```python
from build123d import *

# Parameters (mm, degrees)
SKETCH1_W           = 192.0875
SKETCH1_H           = 95.9358
BOSS_EXTRUDE1_DEPTH = 6.35
SKETCH8_R           = 0.635
CUT_EXTRUDE2_DEPTH  = 20.05
SKETCH3_R           = 2.54
SKETCH3_W           = 12.8016
SKETCH3_H           = 27.94
SKETCH3_W_2         = 18.034
SKETCH3_H_2         = 12.7
CUT_EXTRUDE3_DEPTH  = 7.35


with BuildPart() as part:
    # Sketch1 → Boss-Extrude1 (new body)
    with BuildSketch(Plane(origin=(0, 0, 0), x_dir=(1, 0, 0), z_dir=(0, 1, 0))):
        with Locations((96.04375, 47.9679)):
            Rectangle(SKETCH1_W, SKETCH1_H)
    extrude(amount=BOSS_EXTRUDE1_DEPTH)

    # Sketch8 → Cut-Extrude2 (cut, through all)
    with BuildSketch(Plane.XZ.offset(12.7)):
        with Locations((19.05, 5.6642)):
            Circle(SKETCH8_R)
        with Locations((19.05, 18.3642)):
            Circle(SKETCH8_R)
        with Locations((19.05, -70.5358)):
            Circle(SKETCH8_R)
        with Locations((19.05, -83.2358)):
            Circle(SKETCH8_R)
        with Locations((57.15, -52.7558)):
            Circle(SKETCH8_R)
        with Locations((57.15, -14.6558)):
            Circle(SKETCH8_R)
        with Locations((96.2406, -14.6558)):
            Circle(SKETCH8_R)
        with Locations((96.2406, -52.7558)):
            Circle(SKETCH8_R)
        with Locations((107.95, -83.2358)):
            Circle(SKETCH8_R)
        with Locations((107.95, -70.5358)):
            Circle(SKETCH8_R)
        with Locations((107.95, 5.6642)):
            Circle(SKETCH8_R)
        with Locations((107.95, 18.3642)):
            Circle(SKETCH8_R)
    extrude(amount=-CUT_EXTRUDE2_DEPTH, mode=Mode.SUBTRACT)

    # Sketch3 → Cut-Extrude3 (cut, through all)
    with BuildSketch(Plane(origin=(0, 0, 0), x_dir=(-1, 0, 0), z_dir=(0, -1, 0))):
        with Locations((-96.04375, 25.4)):
            Circle(SKETCH3_R)
        with Locations((-96.04375, 70.5358)):
            Circle(SKETCH3_R)
        with BuildLine():
            Line((-11.43, 88.9508), (-11.43, 82.6008))
            ThreePointArc((-11.43, 82.6008), (-12.7, 81.3308), (-13.97, 82.6008))
            Line((-13.97, 82.6008), (-13.97, 88.9508))
            ThreePointArc((-13.97, 88.9508), (-12.7, 90.2208), (-11.43, 88.9508))
        make_face()
        with BuildLine():
            Line((-182.5625, 84.5058), (-176.2125, 84.5058))
            ThreePointArc((-176.2125, 84.5058), (-174.9425, 85.7758), (-176.2125, 87.0458))
            Line((-176.2125, 87.0458), (-182.5625, 87.0458))
            ThreePointArc((-182.5625, 87.0458), (-183.8325, 85.7758), (-182.5625, 84.5058))
        make_face()
        with BuildLine():
            Line((-9.525, 11.43), (-15.875, 11.43))
            ThreePointArc((-15.875, 11.43), (-17.145, 10.16), (-15.875, 8.89))
            Line((-15.875, 8.89), (-9.525, 8.89))
            ThreePointArc((-9.525, 8.89), (-8.255, 10.16), (-9.525, 11.43))
        make_face()
        with BuildLine():
            Line((-5.1054, 16.7894), (-11.4554, 16.7894))
            ThreePointArc((-11.4554, 16.7894), (-12.5222, 17.8562), (-11.4554, 18.923))
            Line((-11.4554, 18.923), (-5.1054, 18.923))
            ThreePointArc((-5.1054, 18.923), (-4.0386, 17.8562), (-5.1054, 16.7894))
        make_face()
        with BuildLine():
            Line((-186.9821, 16.7894), (-180.6321, 16.7894))
            ThreePointArc((-180.6321, 16.7894), (-179.5653, 17.8562), (-180.6321, 18.923))
            Line((-180.6321, 18.923), (-186.9821, 18.923))
            ThreePointArc((-186.9821, 18.923), (-188.0489, 17.8562), (-186.9821, 16.7894))
        make_face()
        with Locations((-172.5803, 49.1998)):
            Rectangle(SKETCH3_W, SKETCH3_H)
        with Locations((-19.5072, 49.1998)):
            Rectangle(SKETCH3_W, SKETCH3_H)
        with BuildLine():
            Line((-186.9821, 79.1464), (-180.6321, 79.1464))
            ThreePointArc((-180.6321, 79.1464), (-179.5653, 78.0796), (-180.6321, 77.0128))
            Line((-180.6321, 77.0128), (-186.9821, 77.0128))
            ThreePointArc((-186.9821, 77.0128), (-188.0489, 78.0796), (-186.9821, 79.1464))
        make_face()
        with Locations((-75.311, 49.1998)):
            Rectangle(SKETCH3_W_2, SKETCH3_H_2)
    extrude(amount=-CUT_EXTRUDE3_DEPTH, mode=Mode.SUBTRACT)


solid = part.part
```
The listing builds one solid part. Answer for the finished solid, in the listing's coordinates (mm). A direction names the side the tool comes from. Give positions to 0.01 mm unless a question says otherwise; leave off trailing zeros. Write each loop counter-clockwise with the first axis right and the second up, starting at its lowest first coordinate (ties: lowest second). Pieces come first, ordered by that corner, then holes. Notation, with made-up numbers: (-9.5, -5.75) -> (14.5, -5.75) arc R21 ccw to (14.5, 3.25) -> close; hole circle Ø5 at (22, 38). An arc over 180 degrees is marked (long way). Write item = value, one per line. Start each with the question number.
1) The part is cut by section C-C, the plane x = 82. Determine the outline of the cut face in (y, z), and give its area (3 significant figures).
2) The part is cut by section D-D, the plane y = 2. Count the separate pieces of the cut face and the enclosed holes in it, and give its area (3 significant figures).
3) The part is cut by section A-A, the plane z = -61. Determine the outline of the cut face in (x, y).
4) Straight lines are drawn through the part: line 1 along X through (y, z) = (1, -58.5); line 2 along X through (y, z) = (3.75, -49.5); line 3 along Z through (x, y) = (168.5, 1.5). For each, find the intervals that lie inside material, in ascending order.
5) Determine the mould class of faces 3 (the face through (13, 3, -11.43)), 4 (the face through (192.088, 3, -47)), 5 (the face through (95, 3, -95.936)) for opening direction X: +X half, -X half, draft (parallel to the pull), parting line (faces both ways), or undercut.
6) Which of the six approach directions +Z, -Z, +X, -X, +Y, -Y give full straight-line access (tool end or side, diameter ignored) to faces 1 (the face through (0, 3, -47)), 2 (the face through (11.43, 3, -86))?
7) The part is cut by section B-B, the plane z = -25.4. Determine the outline of the cut face in (x, y), and give its area (3 significant figures).
Solutions:
q1.outline = (0, -95.94) -> (6.35, -95.94) -> (6.35, -55.55) -> (0, -55.55) -> close; (0, -42.85) -> (6.35, -42.85) -> (6.35, 0) -> (0, 0) -> close
q1.area = 529 mm²
q2.separate_pieces = 1
q2.enclosed_holes = 19
q2.area = 17,300 mm²
q3.outline = (0, 0) -> (13.11, 0) -> (13.11, 6.35) -> (0, 6.35) -> close; (25.91, 0) -> (166.18, 0) -> (166.18, 6.35) -> (25.91, 6.35) -> close; (178.98, 0) -> (192.09, 0) -> (192.09, 6.35) -> (178.98, 6.35) -> close
q4.line_1 = 0 to 13.11, 25.91 to 166.18, 178.98 to 192.09
q4.line_2 = 0 to 13.11, 25.91 to 66.29, 84.33 to 166.18, 178.98 to 192.09
q4.line_3 = -95.94 to -63.17, -35.23 to 0
q5.face_3 = undercut
q5.face_4 = +X half
q5.face_5 = draft
q6.face_1 = +Z, -Z, -X, +Y, -Y
q6.face_2 = +Y, -Y
q7.outline = (0, 0) -> (93.5, 0) -> (93.5, 6.35) -> (0, 6.35) -> close; (98.58, 0) -> (192.09, 0) -> (192.09, 6.35) -> (98.58, 6.35) -> close
q7.area = 1,190 mm²
